Autodesk Inventor part; units mm, degrees
ref_plane "YZ Plane" through (0, 0, 0) normal (1, 0, 0) x (0, 1, 0)
ref_plane "XZ Plane" through (0, 0, 0) normal (0, 1, 0) x (-1, 0, 0)
ref_plane "XY Plane" through (0, 0, 0) normal (0, 0, 1) x (1, 0, 0)
sketch "Sketch1" plane through (0, 0, 0) normal (0, 0, 1) x (1, 0, 0)
  line L0 (0, 0) -> (60, 0) construction
  circle A0 centre (0, 0) radius 4.5
  circle A1 centre (60, 0) radius 4.5
  line L1 (67.5, -20) -> (-7.5, -20)
  line L2 (-7.5, -20) -> (-7.5, 20)
  line L3 (-7.5, 20) -> (67.5, 20)
  line L4 (67.5, 20) -> (67.5, -20)
  line L5 (67.5, -20) -> (-7.5, 20) construction
  line L6 (-7.5, -20) -> (67.5, 20) construction
  point P0 (30, 0)
  dimension "d0" = 9
  dimension "d1" = 60
  dimension "d2" = 40
  dimension "d3" = 75
extrude "Extrusion1" add sketch "Sketch1" along normal blind 14
sketch "Sketch2" plane through (0, 0, 14) normal (0, 0, 1) x (1, 0, 0)
  line L0 (-7.5, -20) -> (67.5, -20)
  line L1 (24, -20) -> (36, -20)
  line L2 (36, -20) -> (36, -5.7)
  line L3 (36, -5.7) -> (24, -5.7)
  line L4 (24, -5.7) -> (24, -20)
  point P0 (30, -20)
  dimension "d6" = 12
  dimension "d7" = 14.3
extrude "Extrusion2" cut sketch "Sketch2" against normal through all
sketch "Sketch3" plane through (24, -20, 14) normal (1, 0, 0) x (0, 0, -1)
  line L0 (0, 0) -> (8, 0) construction
  line L1 (8, 0) -> (8, 9.5) construction
  line L2 (8, 9.5) -> (0, 9.5) construction
  line L3 (0, 9.5) -> (0, 0) construction
  circle A0 centre (8, 9.5) radius 2.25
  point P0 (14, 20)
  dimension "d10" = 8
  dimension "d11" = 9.5
  dimension "d12" = 4.5
extrude "Extrusion3" cut sketch "Sketch3" along normal through all both and the other way through all
sketch "Sketch4" plane through (0, 0, 14) normal (0, 0, 1) x (1, 0, 0)
  line L0 (67.5, -20) -> (67.5, 20)
  circle A0 centre (0, 0) radius 4.5
  line L1 (-7.5, 20) -> (67.5, 20)
  line L2 (67.5, 20) -> (67.5, 10)
  line L3 (67.5, 10) -> (-7.5, 10)
  line L4 (-7.5, 10) -> (-7.5, 20)
  dimension "d15" = 10
extrude "Extrusion4" cut sketch "Sketch4" against normal through all contours L3 L4 L1 L0
sketch "Sketch5" plane through (0, 0, 0) normal (0, 0, -1) x (-1, 0, 0)
  line L0 (7.5, 10) -> (-67.5, 10)
  line L1 (-45, 10) -> (-15, 10)
  line L2 (-15, 10) -> (-15, 4)
  line L3 (-15, 4) -> (-45, 4)
  line L4 (-45, 4) -> (-45, 10)
  point P0 (-30, 10)
  dimension "d18" = 30
  dimension "d19" = 6
extrude "Extrusion5" cut sketch "Sketch5" against normal through all
chamfer "Chamfer1" distance 6 angle 45 2 edges at (45, 10, 7) (15, 10, 7)
chamfer "Chamfer2" distance 6 angle 45 4 edges at (-7.5, 10, 7) (67.5, 10, 7) (-7.5, -20, 7) (67.5, -20, 7)
properties part number "sensor bracket"
Source: CAD feature listing. Evaluate the final solid. Frame: model axes, mm. A direction names the side the tool comes from. Give positions to 0.01 mm unless a question says otherwise; leave off trailing zeros. Write each loop counter-clockwise with the first axis right and the second up, starting at its lowest first coordinate (ties: lowest second). Pieces come first, ordered by that corner, then holes. Notation, with made-up numbers: (44.25, -23) -> (56.25, -23) arc R33 cw to (56.25, 8) -> close; hole circle Ø9 at (22, 23.5). An arc over 180 degrees is marked (long way). Write item = value, one per line.
Q1. Cut plane D-D on y = 0. Return loops of the section in (x, z), then the cut area to 3 significant figures.
Here are the results:
outline = (-7.5, 0) -> (-4.5, 0) -> (-4.5, 14) -> (-7.5, 14) -> close; (4.5, 0) -> (55.5, 0) -> (55.5, 14) -> (4.5, 14) -> close; (64.5, 0) -> (67.5, 0) -> (67.5, 14) -> (64.5, 14) -> close
area = 798 mm²
Q2. Reachability of faces 5 (the face through (12, 7, 7)), 6 (the face through (36, -13, 7)), 7 (the face through (67.5, -5, 7)) from +Z, -Z, +X, -X, +Y, -Y: full face, straight path, thin tool, end or side. Return the list, or none.
Here are the results:
face_5 = +Z, -Z, +Y
face_6 = +Z, -Z, -Y
face_7 = +Z, -Z, +X, +Y, -Y
Q3. Mould query, pull axis X, two halves, no side actions, for faces 1 (the face through (48, 7, 7)), 2 (the face through (49, -20, 7)), 3 (the face through (-4.5, -17, 7.1)), 4 (the face through (30, -5.7, 7)). Classes: +X half, -X half, draft (parallel to the pull), parting line (faces both ways), or undercut.
Here are the results:
face_1 = undercut
face_2 = draft
face_3 = -X half
face_4 = undercut
Q4. Cut plane C-C on y = -6.5. Return loops of the section in (x, z), then the cut area to 3 significant figures.
Here are the results:
outline = (-7.5, 0) -> (24, 0) -> (24, 14) -> (-7.5, 14) -> close; (36, 0) -> (67.5, 0) -> (67.5, 14) -> (36, 14) -> close
area = 882 mm²
Q5. Cut plane B-B on x = 0. Return loops of the section in (y, z).
Here are the results:
outline = (-20, 0) -> (-4.5, 0) -> (-4.5, 14) -> (-20, 14) -> close; (4.5, 0) -> (10, 0) -> (10, 14) -> (4.5, 14) -> close; hole circle Ø4.5 at (-10.5, 6)
Q6. Line query: line 1 (X direction, y = -7, z = 1.25); line 2 (Y direction, x = 57.5, z = 6.5); line 3 (X direction, y = -3, z = 13.25). Output: solid intervals per line, ascending. Write a range as from..to.
Here are the results:
line_1 = -7.5..24, 36..67.5
line_2 = -20..-12.69, -8.31..-3.74, 3.74..10
line_3 = -7.5..-3.35, 3.35..56.65, 63.35..67.5
Q7. First-contact query: pin 1 (4 mm diameter, centred on y = -10.5, z = 6, fed in from -X); pin 2 (3 mm diameter, centred on x = 21, z = 1.5, fed in from +Y); pin 3 (7 mm diameter, centred on y = -16, z = 6, fed in from -X); pin 4 (1 mm diameter, centred on x = 10.5, z = 9, fed in from +Y). Flat tips, straight axial feed; report the tip coordinate or a pass-through.
Here are the results:
pin_1 = through
pin_2 = 4
pin_3 = -7.5
pin_4 = 9
Q8. Cut plane A-A on z = 6. State how many separate pieces and enclosed holes the cut face has, then the cut area to 3 significant figures.
Here are the results:
separate_pieces = 3
enclosed_holes = 2
area = 1,380 mm²
